Can you work these out from the model? Positions are in its coordinate system, mm. Face numbers are marked on the shaded views. A direction names the side the tool comes from. Give positions to 0.01 mm unless a question says otherwise; leave off trailing zeros. Loops run counter-clockwise (first coordinate to the right, second up) from the corner with the lowest first, then second, coordinate; pieces in that order, holes last. Notation, with made-up numbers: (-16.75, 74) - (2.25, 74) arc R32 ccw to (2.25, 105) - close; hole circle Ø8 at (54, 1). An arc over 180 degrees is marked (long way). Answer as a JSON object with one key per item and string values. Group by question number.
Item 1: Which directions (+Z, -Z, +X, -X, +Y, -Y) give clear straight access to the entire face, cutting with the end or side of a thin tool? Please do the marked faces 1 and 2.
Item 2: Will these pins go through, and if not, where does the flat tip stop? pin 1 (13 mm diameter, centred on x = 0, y = 0, fed in from -Z); pin 2 (12 mm diameter, centred on x = 15, y = -13, fed in from +Z); pin 3 (3 mm diameter, centred on x = 22, y = 14, fed in from +Z); pin 4 (1 mm diameter, centred on x = -7.5, z = 9, fed in from +Y).
Item 3: Suppose I cut it at D-D on z = -9. Write out the boundary of the cut face in (x, y).
Item 4: Suppose I cut it at B-B on x = 0. Write out the boundary of the cut face in (y, z).
Item 5: Suppose I cut it at A-A on y = -7. Write out the boundary of the cut face in (x, z).
Item 6: Please list where these lines run through material, in increasing order: L1, parallel to Z at x = 18, y = -9.5; L2, parallel to X at y = 6, z = 0; L3, parallel to Y at x = 0, z = -16.
Item 7: Suppose I cut it at C-C on z = 6. Write out the boundary of the cut face in (x, y), and give its area (3 significant figures).
from build123d import *

# Parameters (mm, degrees)
SKETCH1_R           = 14
SKETCH1_R_2         = 8
BOSS_EXTRUDE1_DEPTH = 28
SKETCH2_W           = 8
SKETCH2_H           = 56
CUT_EXTRUDE1_START  = -56
SKETCH3_R           = 8
CUT_EXTRUDE1_DEPTH  = 56
CUT_EXTRUDE2_START  = -56
SKETCH4_R           = 8
CUT_EXTRUDE2_DEPTH  = 56


with BuildPart() as part:
    # Sketch1 → Boss-Extrude1 (new, symmetric)
    with BuildSketch(Plane.XY):
        Circle(SKETCH1_R)
        Circle(SKETCH1_R_2, mode=Mode.SUBTRACT)
    extrude(amount=BOSS_EXTRUDE1_DEPTH, both=True)

    # Sketch2 → Revolve1 (revolve)
    with BuildSketch(Plane.XY, mode=Mode.PRIVATE) as revolve1_sk:
        with Locations((30, 0)):
            Rectangle(SKETCH2_W, SKETCH2_H)
    revolve(revolve1_sk.sketch.rotate(Axis((18, -19.968284035, 0), (0, 1, 0)), 90), axis=Axis((18, -19.968284035, 0), (0, 1, 0)))

    # Sketch3 → Cut-Extrude1 (cut)
    with BuildSketch(Plane.XY.offset(28).offset(CUT_EXTRUDE1_START)):
        Circle(SKETCH3_R)
    extrude(amount=CUT_EXTRUDE1_DEPTH, mode=Mode.SUBTRACT)

    # Sketch4 → Cut-Extrude2 (cut)
    with BuildSketch(Plane(origin=(0, 28, 0), x_dir=(1, 0, 0), z_dir=(0, 1, 0)).offset(CUT_EXTRUDE2_START)):
        with Locations(Location((18, 0, 0), (0, 0, 90))):
            Circle(SKETCH4_R)
    extrude(amount=CUT_EXTRUDE2_DEPTH, mode=Mode.SUBTRACT)


solid = part.part
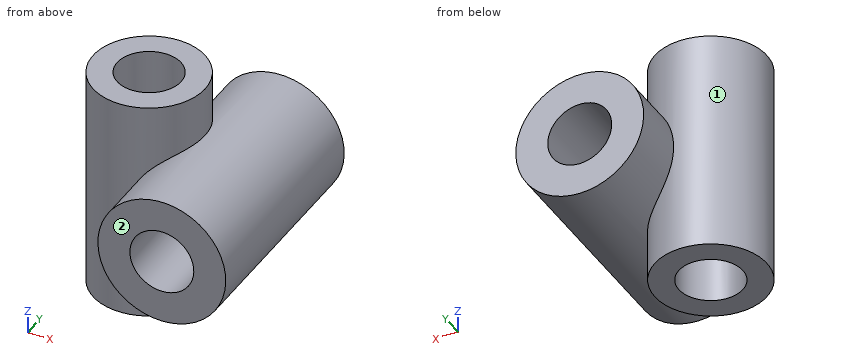
Worked out:
{
 "1": {"face 1": "none", "face 2": "+Z, -Z, +X, -X, -Y"},
 "2": {"pin 1": "passes through", "pin 2": "stops at z = 28", "pin 3": "stops at z = 15.8", "pin 4": "stops at y = 12.12"},
 "3": {"outline": "(4.77, -28) - (31.23, -28) - (31.23, 28) - (4.77, 28) - (4.77, 13.16) arc R14 ccw (long way) to (4.77, -13.16) - close; hole circle Ø16 at (0, 0)"},
 "4": {"outline": "(-14, -28) - (-8, -28) - (-8, 28) - (-14, 28) - close; (8, -28) - (14, -28) - (14, 28) - (8, 28) - close"},
 "5": {"outline": "(-12.12, -28) - (-3.87, -28) - (-3.87, 28) - (-12.12, 28) - close; (3.87, -28) - (12.12, -28) - (12.12, -14.88) arc R16 ccw (long way) to (12.12, 14.88) - (12.12, 28) - (3.87, 28) - close; hole circle Ø16 at (18, 0)"},
 "6": {"L1": "z = -16 to -8, 8 to 16", "L2": "x = -12.65 to -5.29, 5.29 to 10, 26 to 34", "L3": "y = -14 to -8, 8 to 14"},
 "7": {"outline": "(3.17, -28) - (12.71, -28) - (12.71, 28) - (3.17, 28) - (3.17, 13.64) arc R14 ccw (long way) to (3.17, -13.64) - close; (23.29, -28) - (32.83, -28) - (32.83, 28) - (23.29, 28) - close; hole circle Ø16 at (0, 0)", "area": "1,260 mm2"}
}
